Read the model definition and answer for the solid it produces. Units are mm, in the model's axes. Round coordinates to 2 decimals unless told otherwise and drop trailing zeros. Loops run counter-clockwise (first coordinate to the right, second up) from the corner with the lowest first, then second, coordinate; pieces in that order, holes last. Notation, with made-up numbers: M -22,10 L 14,10 A24 ccw 14,28 Z; hole C 64.5,12 d3. An arc over 180 degrees is marked long. Write each question's results on one line, items separated by ' | '.
Autodesk Inventor part; units mm, degrees
ref_plane "YZ Plane" through (0, 0, 0) normal (1, 0, 0) x (0, 1, 0)
ref_plane "XZ Plane" through (0, 0, 0) normal (0, 1, 0) x (-1, 0, 0)
ref_plane "XY Plane" through (0, 0, 0) normal (0, 0, 1) x (1, 0, 0)
sketch "Sketch1" plane through (0, 0, 0) normal (0, 0, 1) x (1, 0, 0)
  line L0 (0, 0) -> (-79.2226, 0)
  line L1 (-79.2226, 0) -> (-79.2226, 12.7)
  line L2 (-79.2226, 12.7) -> (0, 12.7)
  line L3 (0, 12.7) -> (0, 0)
  line L4 (0, 12.7) -> (-29.718, 12.7)
  line L5 (-79.2226, 12.7) -> (-71.7296, 12.7)
  dimension "d1" = 79.2226
  dimension "d2" = 12.7
  dimension "d5" = 7.493
extrude "Plate5" add sketch "Sketch1" along normal blind 3.175
sketch "Sketch6" plane through (3.175, 0, -3.175) normal (1, 0, 0) x (0, 1, 0)
  line L0 (12.7, 0) -> (0, 0)
  line L1 (0, 0) -> (0, -289.3822)
  line L2 (0, -289.3822) -> (12.7, -289.3822)
  line L3 (12.7, -289.3822) -> (12.7, 0)
edge flange "Flange4" height 295.7322 angle 90 thickness 3.175 bend radius 3.175 thickness toward (1, 0, 0) relief tear relief width 3.175 relief depth 1.5875 edges at (0, 6.35, 0) wall of the first edge with corners at (3.175, 12.7, -3.175) (3.175, 0, -3.175) (3.175, 0, -292.5572) (3.175, 12.7, -292.5572)
bend "Bend4"
corner "Corner4"
sketch "Sketch7" plane through (0, 0, -295.7322) normal (0, 0, -1) x (-1, 0, 0)
  line L0 (0, 12.7) -> (0, 0)
  line L1 (0, 0) -> (79.2226, 0)
  line L2 (79.2226, 0) -> (79.2226, 12.7)
  line L3 (79.2226, 12.7) -> (0, 12.7)
edge flange "Flange5" height 85.5726 angle 90 thickness 3.175 bend radius 3.175 thickness toward (0, 0, -1) relief tear relief width 3.175 relief depth 1.5875 edges at (3.175, 6.35, -292.5572) wall of the first edge with corners at (0, 12.7, -295.7322) (0, 0, -295.7322) (-79.2226, 0, -295.7322) (-79.2226, 12.7, -295.7322)
bend "Bend5"
corner "Corner5"
sketch "Sketch8" plane through (0, 0, 3.175) normal (0, 0, 1) x (1, 0, 0)
  circle A0 centre (-71.725, 5.9188) radius 3.3
  circle A1 centre (-29.725, 5.9188) radius 3.3
extrude "Extrusion2" cut sketch "Sketch8" against normal blind 2539974.6
equation "\"d43\" = BendReliefWidth"
equation "\"d44\" = BendReliefDepth"
equation "\"d45\" = MinimumRemnant"
equation "\"d46\" = BendRadius"
equation "\"d49\" = BendRadius"
equation "\"d50\" = CornerReliefSize"
equation "\"d51\" = GapSize"
equation "\"d52\" = JacobiRadiusSize"
equation "\"d53\" = BendReliefWidth"
equation "\"d54\" = BendReliefDepth"
equation "\"d55\" = MinimumRemnant"
equation "\"d56\" = BendRadius"
equation "\"d59\" = BendRadius"
equation "\"d60\" = CornerReliefSize"
equation "\"d61\" = GapSize"
equation "\"d62\" = JacobiRadiusSize"
equation "\"BendRadius\" = Thickness"
equation "\"BendReliefWidth\" = Thickness"
equation "\"BendReliefDepth\" = 0.5 * Thickness"
equation "\"CornerReliefSize\" = 4 * Thickness"
equation "\"MinimumRemnant\" = 2 * Thickness"
equation "\"TransitionRadius\" = BendRadius"
equation "\"JacobiRadiusSize\" = BendRadius"
equation "\"GapSize\" = Thickness"
equation "\"d8\" = BendRadius"
equation "\"d42\" = BendRadius"
properties part number "tie-together tier 2 wide" material "Aluminum 6061"
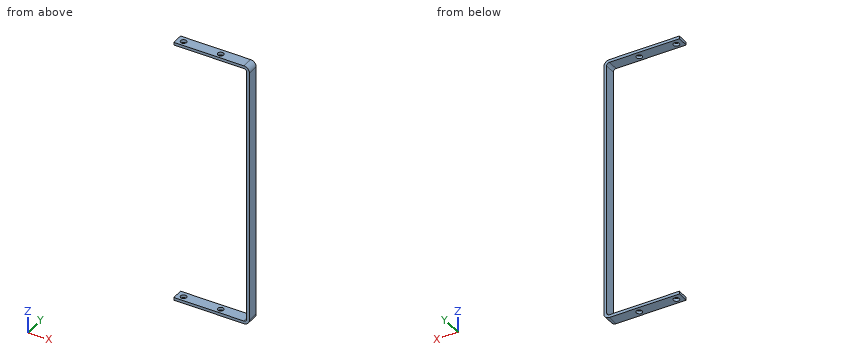
Item 1: The part is cut by section A-A (x = -21). Determine the outline of the cut face in (y, z) (3 decimals), plus the area to 3 significant figures.
Outcome:
outline: M 0,-298.907 L 12.7,-298.907 L 12.7,-295.732 L 0,-295.732 Z; M 0,0 L 12.7,0 L 12.7,3.175 L 0,3.175 Z | area: 80.6 mm2
Item 2: Straight lines are drawn through the part: line 1 (Z direction, x = -25, y = 6.5) (3 decimals); line 2 (X direction, y = 11.25, z = -47.5) (3 decimals). For each, find the intervals that lie inside material, in ascending order.
Outcome:
line 1: z = -298.907 to -295.732, 0 to 3.175 | line 2: x = 3.175 to 6.35
Item 3: The part is cut by section B-B (z = -203). Determine the outline of the cut face in (x, y) (3 decimals), plus the area to 3 significant figures.
Outcome:
outline: M 3.175,0 L 6.35,0 L 6.35,12.7 L 3.175,12.7 Z | area: 40.3 mm2
